For this review, take the finished solid that the model builds, in its own axes (mm). Face numbers are marked on the shaded views. A direction names the side the tool comes from. Coordinates: 2 decimals unless noted, no trailing zeros. Write each loop counter-clockwise with the first axis right and the second up, starting at its lowest first coordinate (ties: lowest second). Pieces come first, ordered by that corner, then holes. Notation, with made-up numbers: M 46,69.5 L 59,69.5 A20 cw 59,103.5 Z; hole C 55.25,75.25 d7. An arc over 180 degrees is marked long. One line per question, with ' | ' between items.
from build123d import *

# Parameters (mm, degrees)
PAD_DEPTH   = 25
SKETCH001_R = 2.5
HOLE_DEPTH  = 45


with BuildPart() as part:
    # Sketch → Pad (new body)
    with BuildSketch(Plane.XZ):
        Polygon((-21, -19.977354), (21, -19.977354), (21, -14.977354), (6, -14.977354), (6, 15.022646), (21, 15.022646), (21, 20.022646), (-1, 20.022646), (-1, -4.977354), (-21, -4.977354), align=None)
    extrude(amount=PAD_DEPTH)

    # Sketch001 (on Face6 of Pad) → Hole (cut)
    with BuildSketch(Plane(origin=(21, 0, 0), x_dir=(0, 0, 1), z_dir=(1, 0, 0))):
        with Locations((-10.960537, 18.936941)):
            Circle(SKETCH001_R)
        with Locations((-11.072524, 5.050469)):
            Circle(SKETCH001_R)
    extrude(amount=-HOLE_DEPTH, mode=Mode.SUBTRACT)


solid = part.part
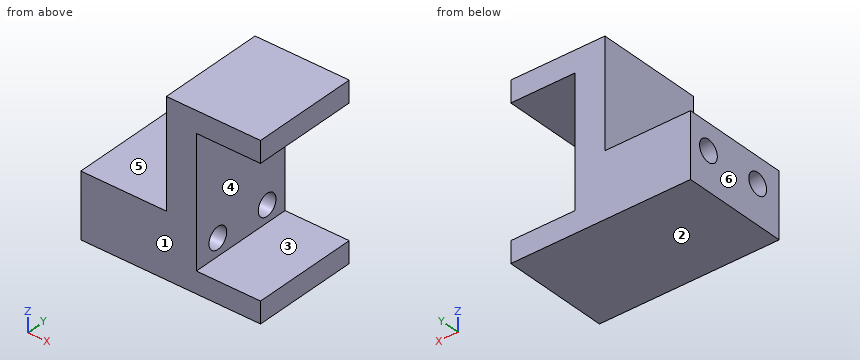
1) We need section B-B on y = -19.75. State the section outline as (x, z) points.
Responses:
outline: M -21,-19.98 L 21,-19.98 L 21,-14.98 L 6,-14.98 L 6,-13.32 L -21,-13.32 Z; M -21,-8.6 L 6,-8.6 L 6,15.02 L 21,15.02 L 21,20.02 L -1,20.02 L -1,-4.98 L -21,-4.98 Z
2) We need section C-C on z = -12.5. State the section outline as (x, y) points.
Responses:
outline: M -21,-25 L 6,-25 L 6,-20.91 L -21,-20.91 Z; M -21,-16.97 L 6,-16.97 L 6,-7.1 L -21,-7.1 Z; M -21,-3 L 6,-3 L 6,0 L -21,0 Z
3) Machinability: for the marked faces 4, 5 and 6, which of the approach directions +Z, -Z, +X, -X, +Y, -Y give a long, thin tool a straight path to every point of the face, cutting with its end or side? Answer none if there is none.
Responses:
face 4: +X, +Y, -Y | face 5: +Z, -X, +Y, -Y | face 6: +Z, -Z, -X, +Y, -Y
4) To check wall thickness, follow line 1 along Z through (x, y) = (12, -3.75); line 2 along Z through (x, y) = (3.5, -5); line 3 along X through (y, z) = (-23.25, -4). State the ranges of each line that lie inside material, in increasing order. Write a range as [from, to].
Responses:
line 1: [-19.98, -14.98], [15.02, 20.02] | line 2: [-19.98, -13.57], [-8.57, 20.02] | line 3: [-1, 6]
5) Insertion check: pin 1 Ø10 at (x, y) = (-7, -13.5) entering from +Z; pin 2 Ø6 at (x, z) = (-6.5, 7.5) entering from -Y; pin 3 Ø12.5 at (y, z) = (-6.5, -3.5) entering from +X. Each pin has a flat end and moves straight along its axis. Give the tip position at first contact, or say it passes through.
Responses:
pin 1: z = -4.98 | pin 2: through | pin 3: x = 6
6) The part is to be moulded in two halves that separate along Z. For the marked faces 1, 2 and 3, say which applies: +Z half, -Z half, draft (parallel to the pull), parting line (faces both ways), or undercut.
Responses:
face 1: draft | face 2: -Z half | face 3: undercut
7) We need section D-D on y = -22.75. State the section outline as (x, z) points, then the cut area to 3 significant figures.
Responses:
outline: M -21,-19.98 L 21,-19.98 L 21,-14.98 L 6,-14.98 L 6,15.02 L 21,15.02 L 21,20.02 L -1,20.02 L -1,-4.98 L -21,-4.98 Z | area: 730 mm^2
8) We need section A-A on x = 9.5. State the section outline as (y, z) points, then the cut area to 3 significant figures.
Responses:
outline: M -25,-19.98 L 0,-19.98 L 0,-14.98 L -25,-14.98 Z; M -25,15.02 L 0,15.02 L 0,20.02 L -25,20.02 Z | area: 250 mm^2
